Can you work these out from the model? Positions are in its coordinate system, mm. A direction names the side the tool comes from. Round coordinates to 2 decimals unless told otherwise and drop trailing zeros. Write each loop counter-clockwise with the first axis right and the second up, starting at its lowest first coordinate (ties: lowest second). Pieces come first, ordered by that corner, then holes. Notation, with made-up numbers: M 33,40 L 72,40 A18 ccw 72,63 Z; hole C 31.25,-29 d4. An arc over 180 degrees is marked long. Use one line per item in the form item = value. Start each with the question number.
```python
from build123d import *

# Parameters (mm, degrees)
SKETCH1_W           = 185
SKETCH1_H           = 142
BOSS_EXTRUDE1_DEPTH = 23
SKETCH12_W          = 80
SKETCH12_H          = 100
BOSS_EXTRUDE6_DEPTH = 53
SHELL1_T            = -5
SKETCH11_R          = 6.25
CUT_EXTRUDE2_DEPTH  = 6
FILLET1_R           = 2
SKETCH13_R          = 1.95
CUT_EXTRUDE3_DEPTH  = 54


with BuildPart() as part:
    # Sketch1 → Boss-Extrude1 (new body)
    with BuildSketch(Plane(origin=(0, 0, 0), x_dir=(1, 0, 0), z_dir=(0, 1, 0))):
        with Locations((92.5, 71)):
            Rectangle(SKETCH1_W, SKETCH1_H)
    extrude(amount=BOSS_EXTRUDE1_DEPTH)

    # Sketch12 → Boss-Extrude6 (add)
    with BuildSketch(Plane(origin=(0, 0, 0), x_dir=(1, 0, 0), z_dir=(0, 1, 0))):
        with Locations((40, 140)):
            Rectangle(SKETCH12_W, SKETCH12_H)
    extrude(amount=BOSS_EXTRUDE6_DEPTH)

    # Shell1
    shell1_openings = [part.faces().sort_by_distance(p)[0] for p in [
        (88.333333333, 0, -110.666666667),
        (185, 11.5, -71),
        (0, 25.333333333, -93.333333333),
    ]]
    offset(amount=SHELL1_T, openings=shell1_openings, kind=Kind.INTERSECTION)

    # Sketch11 → Cut-Extrude2 (cut)
    with BuildSketch(Plane.XY):
        with Locations((18.4375, 9.5)):
            Circle(SKETCH11_R)
        with Locations((43.088852194, 9.5)):
            Circle(SKETCH11_R)
        with Locations((67.740204388, 9.5)):
            Circle(SKETCH11_R)
        with Locations((92.391556582, 9.5)):
            Circle(SKETCH11_R)
        with Locations((117.042908776, 9.5)):
            Circle(SKETCH11_R)
        with Locations((141.69426097, 9.5)):
            Circle(SKETCH11_R)
        with Locations((166.345613164, 9.5)):
            Circle(SKETCH11_R)
    extrude(amount=-CUT_EXTRUDE2_DEPTH, mode=Mode.SUBTRACT)

    # Fillet1
    fillet1_edges = [part.edges().sort_by_distance(p)[0] for p in [
        (92.5, 18, -5),
        (130, 18, -137),
        (37.5, 48, -95),
        (75, 48, -140),
        (37.5, 48, -185),
    ]]
    fillet(fillet1_edges, radius=FILLET1_R)

    # Sketch13 → Cut-Extrude3 (cut, through all)
    with BuildSketch(Plane(origin=(0, 53, 0), x_dir=(1, 0, 0), z_dir=(0, 1, 0))):
        with Locations((15, 100.5)):
            Circle(SKETCH13_R)
        with Locations((15, 179.5)):
            Circle(SKETCH13_R)
        with Locations((65, 179.5)):
            Circle(SKETCH13_R)
        with Locations((65, 100.5)):
            Circle(SKETCH13_R)
    extrude(amount=-CUT_EXTRUDE3_DEPTH, mode=Mode.SUBTRACT)


solid = part.part
```
1. If we section it at B-B (x = 57): List the corners of the cut face in (y, z) for me, and give its area (3 significant figures).
2. If we section it at D-D (y = 9.5): State how many separate pieces and enclosed holes the cut face has, and give its area (3 significant figures).
3. If we mould it in two halves opening along Y, with no side actions, what happens to faces 5 (the face through (13.478, 5.697, -2.465)), 6 (the face through (132, 11, -142)), 7 (the face through (39, 53, -141))? For each: pulls with the +Y half, pulls with the -Y half, needs draft (parallel to the pull), parting line crosses it, or undercut.
4. Please list where these lines run through material, in increasing order: line 1 along X through (y, z) = (51.15, -179.5); line 2 along Z through (x, y) = (15, 49); line 3 along Z through (x, y) = (70.5, 39).
5. If we section it at A-A (y = 35): List the corners of the cut face in (x, z) for me.
6. Will these pins go through, and if not, where does the flat tip stop? pin 1 (20 mm diameter, centred on x = 166.35, y = 9.5, fed in from -Z); pin 2 (10 mm diameter, centred on x = 32, z = -20.5, fed in from -Y); pin 3 (10 mm diameter, centred on x = 58, y = 41.5, fed in from +Z).
7. Which directions (+Z, -Z, +X, -X, +Y, -Y) give clear straight access to the entire face, cutting with the end or side of a thin tool? Please do faces 1 (the face through (87.43, 5.7, -2.46)), 2 (the face through (91, 3, -5)), 3 (the face through (36, 48, -141)), 4 (the face through (39, 26, -190)).
8. If we section it at C-C (x = 20.5): List the corners of the cut face in (y, z) for me, and give its area (3 significant figures).
Model answer:
q1.outline = M 0,-190 L 53,-190 L 53,-90 L 23,-90 L 23,0 L 0,0 L 0,-5 L 16,-5 A2 cw 18,-7 L 18,-95 L 46,-95 A2 cw 48,-97 L 48,-183 A2 cw 46,-185 L 0,-185 Z
q1.area = 1,430 mm2
q2.separate_pieces = 9
q2.enclosed_holes = 0
q2.area = 1,650 mm2
q3.face_5 = undercut
q3.face_6 = needs draft
q3.face_7 = pulls with the +Y half
q4.line_1 = 0 to 13.05, 16.95 to 63.05, 66.95 to 80
q4.line_2 = -190 to -181.45, -177.55 to -102.45, -98.55 to -90
q4.line_3 = -190 to -185, -95 to -90
q5.outline = M 0,-190 L 80,-190 L 80,-90 L 0,-90 L 0,-95 L 75,-95 L 75,-185 L 0,-185 Z
q6.pin_1 = -142
q6.pin_2 = 18
q6.pin_3 = -90
q7.face_1 = +Z
q7.face_2 = +X, -X, -Y
q7.face_3 = -X, -Y
q7.face_4 = -Z, +X, -X, +Y, -Y
q8.outline = M 0,-190 L 53,-190 L 53,-90 L 23,-90 L 23,0 L 15.4,0 L 15.4,-5 L 16,-5 A2 cw 18,-7 L 18,-95 L 46,-95 A2 cw 48,-97 L 48,-183 A2 cw 46,-185 L 0,-185 Z; M 0,-5 L 3.6,-5 L 3.6,0 L 0,0 Z
q8.area = 1,370 mm2
